Source: three-view drawing plus pictorial views. Frame: mm from the lowest corner of the part. Give positions to 0.01 mm unless a question says otherwise; leave off trailing zeros. Loops run counter-clockwise (first coordinate to the right, second up) from the corner with the lowest first, then second, coordinate; pieces in that order, holes last.
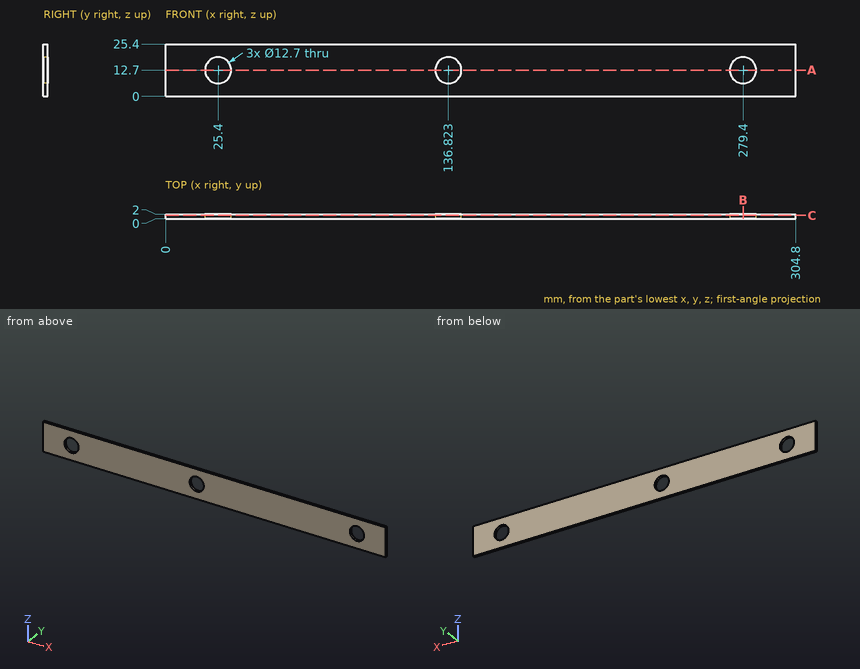
(1) Cut plane B-B (x = 279.4). Return the cut outline in (y, z).
Values follow:
outline: (0, 0) - (2, 0) - (2, 6.35) - (0, 6.35) - close; (0, 19.05) - (2, 19.05) - (2, 25.4) - (0, 25.4) - close
(2) Cut plane C-C (y = 1.6). Return the cut outline in (x, z), and give its area (3 significant figures).
Values follow:
outline: (0, 0) - (304.8, 0) - (304.8, 25.4) - (0, 25.4) - close; hole circle Ø12.7 at (25.4, 12.7); hole circle Ø12.7 at (136.82, 12.7); hole circle Ø12.7 at (279.4, 12.7)
area: 7,360 mm2
(3) Pin query (flat end, axial travel): pin 1 Ø10 at (x, z) = (279.4, 12.7) entering from -Y. Return the tip coordinate at first contact, or that it passes through.
Values follow:
pin 1: passes through
(4) Ray query, probe 1 along X at (y, z) = (1.95, 13.25); probe 2 along X at (y, z) = (1.7, 13); probe 3 along Z at (x, y) = (25.4, 0.9). Return the intervals inside material, ascending.
Values follow:
probe 1: x = 0 to 19.07, 31.73 to 130.5, 143.15 to 273.07, 285.73 to 304.8
probe 2: x = 0 to 19.06, 31.74 to 130.48, 143.17 to 273.06, 285.74 to 304.8
probe 3: z = 0 to 6.35, 19.05 to 25.4
(5) Cut plane A-A (z = 12.7). Return the cut outline in (x, y).
Values follow:
outline: (0, 0) - (19.05, 0) - (19.05, 2) - (0, 2) - close; (31.75, 0) - (130.47, 0) - (130.47, 2) - (31.75, 2) - close; (143.17, 0) - (273.05, 0) - (273.05, 2) - (143.17, 2) - close; (285.75, 0) - (304.8, 0) - (304.8, 2) - (285.75, 2) - close
